```python
from build123d import *

# Parameters (mm, degrees)
SKETCH1_W           = 56.22
SKETCH1_H           = 56.22
BOSS_EXTRUDE1_DEPTH = 4.9
SKETCH2_R           = 2.5
CUT_EXTRUDE1_DEPTH  = 5.9
FILLET1_R           = 2
BOSS_EXTRUDE2_DEPTH = 49.81
FILLET2_R           = 2
SKETCH5_R           = 19.035
BOSS_EXTRUDE3_DEPTH = 1.6
SKETCH6_R           = 3.175
BOSS_EXTRUDE4_DEPTH = 19.37


with BuildPart() as part:
    # Sketch1 → Boss-Extrude1 (new body)
    with BuildSketch(Plane.XY):
        with Locations((28.11, 28.11)):
            Rectangle(SKETCH1_W, SKETCH1_H)
    extrude(amount=BOSS_EXTRUDE1_DEPTH)

    # Sketch2 → Cut-Extrude1 (cut, through all)
    with BuildSketch(Plane(origin=(0, 0, 0), x_dir=(-1, 0, 0), z_dir=(0, 0, -1))):
        with Locations((-4.6, 51.62)):
            Circle(SKETCH2_R)
        with Locations((-51.62, 51.62)):
            Circle(SKETCH2_R)
        with Locations((-51.62, 4.6)):
            Circle(SKETCH2_R)
        with Locations((-4.6, 4.6)):
            Circle(SKETCH2_R)
    extrude(amount=-CUT_EXTRUDE1_DEPTH, mode=Mode.SUBTRACT)

    # Fillet1
    fillet1_edges = [part.edges().sort_by_distance(p)[0] for p in [
        (0, 56.22, 2.45),
        (56.22, 56.22, 2.45),
        (56.22, 0, 2.45),
        (0, 0, 2.45),
    ]]
    fillet(fillet1_edges, radius=FILLET1_R)

    # Sketch4 → Boss-Extrude2 (add)
    with BuildSketch(Plane.XY.offset(4.9)):
        Polygon((0, 46.22), (0, 28.11), (28.11, 28.11), (28.11, 56.22), (10, 56.22), (10, 46.22), align=None)
        Polygon((28.11, 56.22), (28.11, 28.11), (56.22, 28.11), (56.22, 46.22), (46.22, 46.22), (46.22, 56.22), align=None)
        Polygon((56.22, 28.11), (28.11, 28.11), (28.11, 0), (46.22, 0), (46.22, 10), (56.22, 10), align=None)
        Polygon((28.11, 28.11), (0, 28.11), (0, 10), (10, 10), (10, 0), (28.11, 0), align=None)
    extrude(amount=BOSS_EXTRUDE2_DEPTH)

    # Fillet2
    fillet2_edges = [part.edges().sort_by_distance(p)[0] for p in [
        (10, 0, 29.805),
        (46.22, 0, 29.805),
        (46.22, 10, 29.805),
        (56.22, 10, 29.805),
        (56.22, 46.22, 29.805),
        (46.22, 46.22, 29.805),
        (46.22, 56.22, 29.805),
        (10, 56.22, 29.805),
        (10, 46.22, 29.805),
        (0, 46.22, 29.805),
        (0, 10, 29.805),
        (10, 10, 29.805),
    ]]
    fillet(fillet2_edges, radius=FILLET2_R)

    # Sketch5 → Boss-Extrude3 (add)
    with BuildSketch(Plane(origin=(0, 0, 0), x_dir=(-1, 0, 0), z_dir=(0, 0, -1))):
        with Locations((-28.11, 28.11)):
            Circle(SKETCH5_R)
    extrude(amount=BOSS_EXTRUDE3_DEPTH)

    # Sketch6 → Boss-Extrude4 (add)
    with BuildSketch(Plane(origin=(0, 0, -1.6), x_dir=(-1, 0, 0), z_dir=(0, 0, -1))):
        with Locations((-28.11, 28.11)):
            Circle(SKETCH6_R)
    extrude(amount=BOSS_EXTRUDE4_DEPTH)


solid = part.part
```
Geometry: final body of the model. Coordinates: model frame, mm. A direction names the side the tool comes from. Round coordinates to 2 decimals unless told otherwise and drop trailing zeros. Write each loop counter-clockwise with the first axis right and the second up, starting at its lowest first coordinate (ties: lowest second). Pieces come first, ordered by that corner, then holes. Notation, with made-up numbers: (58.25, -3.75) -> (76.25, -3.75) arc R28 cw to (76.25, 14.25) -> close; hole circle Ø2 at (29, 56.25). An arc over 180 degrees is marked (long way). Return JSON: item names as keys, results as strings.
Q1. Section A-A on x = 51.62. Return the cut outline in (y, z), and give its area (3 significant figures).
From the geometry:
{"outline": "(0, 0) -> (2.1, 0) -> (2.1, 4.9) -> (0, 4.9) -> close; (7.1, 0) -> (49.12, 0) -> (49.12, 4.9) -> (46.22, 4.9) -> (46.22, 54.71) -> (10, 54.71) -> (10, 4.9) -> (7.1, 4.9) -> close; (54.12, 0) -> (56.22, 0) -> (56.22, 4.9) -> (54.12, 4.9) -> close", "area": "2,030 mm2"}
Q2. Mould query, pull axis Y, two halves, no side actions, for faces 4 (the flat face through (49, 5, 4.9)), 5 (the cylindrical face through (5.14, 49.18, 2.42)), 6 (the cylindrical face through (45.62, 0.57, 30.15)). Classes: +Y half, -Y half, draft (parallel to the pull), parting line (faces both ways), or undercut.
From the geometry:
{"face 4": "draft", "face 5": "undercut", "face 6": "-Y half"}
Q3. Set-up query: faces 1 (the cylindrical face through (55.65, 45.62, 30.15)), 2 (the cylindrical face through (9.4, 46.79, 30.15)), 3 (the cylindrical face through (10.6, 0.57, 30.15)). Return all of +Z, -Z, +X, -X, +Y, -Y with unobstructed straight access to the full face (end or side cutting, diameter ignored); none if empty.
From the geometry:
{"face 1": "+Z, +X, +Y", "face 2": "+Z, -X, +Y", "face 3": "+Z, -X, -Y"}
Q4. Section C-C on z = 47.5. Return the cut outline in (x, y), and give its area (3 significant figures).
From the geometry:
{"outline": "(0, 12) arc R2 ccw to (2, 10) -> (8, 10) arc R2 cw to (10, 8) -> (10, 2) arc R2 ccw to (12, 0) -> (44.22, 0) arc R2 ccw to (46.22, 2) -> (46.22, 8) arc R2 cw to (48.22, 10) -> (54.22, 10) arc R2 ccw to (56.22, 12) -> (56.22, 44.22) arc R2 ccw to (54.22, 46.22) -> (48.22, 46.22) arc R2 cw to (46.22, 48.22) -> (46.22, 54.22) arc R2 ccw to (44.22, 56.22) -> (12, 56.22) arc R2 ccw to (10, 54.22) -> (10, 48.22) arc R2 cw to (8, 46.22) -> (2, 46.22) arc R2 ccw to (0, 44.22) -> close", "area": "2,760 mm2"}
Q5. First-contact query: pin 1 Ø6.5 at (x, y) = (4.6, 51.62) entering from -Z; pin 2 Ø5 at (y, z) = (51.5, 23.5) entering from +X; pin 3 Ø6.5 at (x, y) = (4.6, 4.6) entering from +Z; pin 4 Ø4.5 at (x, y) = (51.62, 51.62) entering from +Z. Flat tips, straight axial feed; report the tip coordinate or a pass-through.
From the geometry:
{"pin 1": "z = 0", "pin 2": "x = 46.22", "pin 3": "z = 4.9", "pin 4": "through"}
Q6. Ray query, line 1 (Y direction, x = 4.6, z = 1.5); line 2 (Z direction, x = 19, y = 16); line 3 (Y direction, x = 4, z = 1). Return the intervals inside material, ascending.
From the geometry:
{"line 1": "0 to 2.1, 7.1 to 49.12, 54.12 to 56.22", "line 2": "-1.6 to 54.71", "line 3": "0 to 2.17, 7.03 to 49.19, 54.05 to 56.22"}
Q7. Section D-D on y = 28.11. Return the cut outline in (x, z) (3 decimals), and give its area (3 significant figures).
From the geometry:
{"outline": "(0, 0) -> (9.075, 0) -> (9.075, -1.6) -> (24.935, -1.6) -> (24.935, -20.97) -> (31.285, -20.97) -> (31.285, -1.6) -> (47.145, -1.6) -> (47.145, 0) -> (56.22, 0) -> (56.22, 54.71) -> (0, 54.71) -> close", "area": "3,260 mm2"}
